```python
from build123d import *

# Parameters (mm, degrees)
ESQUISSE1_R                               = 12.5
BOSS_EXTRU_1_DEPTH                        = 1
BOSS_EXTRU_2_DEPTH                        = 1
TROU_POUR_TARAUDAGE_POUR_TROU_TARAUD_M5_D = 4.2
ESQUISSE8_R                               = 3.25
ENL_V_MAT_EXTRU_1_DEPTH                   = 2
CONG_1_R                                  = 10


with BuildPart() as part:
    # Esquisse1 → Boss.-Extru.1 (new body)
    with BuildSketch(Plane.XY):
        Circle(ESQUISSE1_R)
    extrude(amount=BOSS_EXTRU_1_DEPTH)

    # Esquisse4 → Boss.-Extru.2 (add)
    with BuildSketch(Plane.XY.offset(1)):
        with BuildLine():
            Line((-26, 7.00382031), (-10.353574313, 7.00382031))
            ThreePointArc((-10.353574313, 7.00382031), (-12.5, 0), (-10.353574313, -7.00382031))
            Line((-10.353574313, -7.00382031), (-26, -7.00382031))
            ThreePointArc((-26, -7.00382031), (-33.00382031, 0), (-26, 7.00382031))
        make_face()
    extrude(amount=-BOSS_EXTRU_2_DEPTH)

    # Trou pour taraudage pour trou taraudé M52 (through all)
    with Locations(Plane.XY.offset(1)):
        with Locations((-26, 0)):
            Hole(TROU_POUR_TARAUDAGE_POUR_TROU_TARAUD_M5_D / 2)

    # Esquisse8 → Enlèv. mat.-Extru.1 (cut, through all)
    with BuildSketch(Plane(origin=(0, 0, 0), x_dir=(-1, 0, 0), z_dir=(0, 0, -1))):
        Circle(ESQUISSE8_R)
    extrude(amount=-ENL_V_MAT_EXTRU_1_DEPTH, mode=Mode.SUBTRACT)

    # Congé1
    cong_1_edges = [part.edges().sort_by_distance(p)[0] for p in [
        (-10.353574313, 7.00382031, 0.5),
        (-10.353574313, -7.00382031, 0.5),
    ]]
    fillet(cong_1_edges, radius=CONG_1_R)


solid = part.part
```
The model under review builds one solid part; all positions refer to its coordinate system, in mm. A direction names the side the tool comes from. Round coordinates to 2 decimals unless told otherwise and drop trailing zeros. Write each loop counter-clockwise with the first axis right and the second up, starting at its lowest first coordinate (ties: lowest second). Pieces come first, ordered by that corner, then holes.
(1) We need section C-C on y = 0. Give the boundary of the cut face in (x, z).
(2) Insertion check: pin 1 (0.5 mm diameter, centred on x = -17.5, z = 0.5, fed in from +Y); pin 2 (2 mm diameter, centred on x = -17.5, y = 8.5, fed in from +Z). Each pin has a flat end and moves straight along its axis. Give the tip position at first contact, or say it passes through.
(3) We need section A-A on x = 0. Give the boundary of the cut face in (y, z).
(4) Mouldability with a two-part tool opening along Y and no side actions: class faces 1 (the cylindrical face through (2.579, -1.978, 0.493)), 2 (the flat face through (-20.3, -7.004, 0.5)), 3 (the flat face through (-6, 0, 0)) as +Y half, -Y half, draft (parallel to the pull), parting line (faces both ways), or undercut.
(5) We need section D-D on x = -19. Give the boundary of the cut face in (y, z), and give its area (3 significant figures).
(6) Machinability: for faces 4 (the flat face through (-20.4, 7.004, 0.5)), 5 (the cylindrical face through (12.494, -0.4, 0.493)), which of the approach directions +Z, -Z, +X, -X, +Y, -Y give a long, thin tool a straight path to every point of the face, cutting with its end or side? Answer none if there is none.
(7) Wall thickness on L1, parallel to Y at x = -26, z = 0.7; L2, parallel to Y at x = 0, z = 0.65; L3, parallel to X at y = 0.5, z = 0.9: over which ranges is each line inside the solid? List them lowest first.
(8) We need section B-B on z = 0.4. Give the boundary of the cut face in (x, y) (3 decimals), and give its area (3 significant figures).
Findings below:
1. outline: (-33, 0) - (-28.1, 0) - (-28.1, 1) - (-33, 1) - close; (-23.9, 0) - (-3.25, 0) - (-3.25, 1) - (-23.9, 1) - close; (3.25, 0) - (12.5, 0) - (12.5, 1) - (3.25, 1) - close
2. pin 1: stops at y = 7
2. pin 2: passes through
3. outline: (-12.5, 0) - (-3.25, 0) - (-3.25, 1) - (-12.5, 1) - close; (3.25, 0) - (12.5, 0) - (12.5, 1) - (3.25, 1) - close
4. face 1: undercut
4. face 2: -Y half
4. face 3: draft
5. outline: (-7, 0) - (7, 0) - (7, 1) - (-7, 1) - close
5. area: 14.0 mm2
6. face 4: +Z, -Z, -X, +Y
6. face 5: +Z, -Z
7. L1: y = -7 to -2.1, 2.1 to 7
7. L2: y = -12.5 to -3.25, 3.25 to 12.5
7. L3: x = -32.99 to -28.04, -23.96 to -3.21, 3.21 to 12.49
8. outline: (-26, -7.004) - (-14.735, -7.004) arc R10 cw to (-8.186, -9.447) arc R12.5 ccw (long way) to (-8.186, 9.447) arc R10 cw to (-14.735, 7.004) - (-26, 7.004) arc R7.004 ccw to start; hole circle Ø4.2 at (-26, 0); hole circle Ø6.5 at (0, 0)
8. area: 724 mm2
